Model file for the job. Use its own axes, mm. Face numbers are marked on the shaded views. A direction names the side the tool comes from. Coordinates: 2 decimals unless noted, no trailing zeros. Write each loop counter-clockwise with the first axis right and the second up, starting at its lowest first coordinate (ties: lowest second). Pieces come first, ordered by that corner, then holes. Notation, with made-up numbers: M 44,89.5 L 62,89.5 A23 cw 62,121.5 Z; hole C -18.5,9 d11. An arc over 180 degrees is marked long. Put each result on its own line as item: value. Start each with the question number.
Q1. Drop flat-ended pins along their axis: pin 1 (1.5 mm diameter, centred on y = 2, z = 4.5, fed in from +X); pin 2 (1.5 mm diameter, centred on y = -1, z = 6, fed in from -X); pin 3 (4 mm diameter, centred on x = 7.5, z = 5, fed in from +Y). Give the stop position or say it passes through.
Q2. Drill centre lines: line 1 along Y through (x, z) = (0, 3.75); line 2 along Y through (x, z) = (8.5, 6); line 3 along X through (y, z) = (0.75, 5). Where is each one in solid material? Low to high.
Q3. Cut at A-A (y = 0). Write the cut outline in (x, z), then the cut area to 3 significant figures.
Q4. Cut at D-D (y = 2.5). Write the cut outline in (x, z).
Q5. Cut at C-C (x = -0.75). Write the cut outline in (y, z).
Q6. Which spindle directions (+Z, -Z, +X, -X, +Y, -Y) get a long thin tool onto all of the face, cutting with end or side? Do the marked faces 1, 2 and 3. Say none if no direction does.
Q7. Cut at B-B (z = 6.25). Write the cut outline in (x, y).
```python
from build123d import *

# Parameters (mm, degrees)
CROQUIS1_R              = 4
CROQUIS1_R_2            = 2
SALIENTE_EXTRUIR1_DEPTH = 8
CROQUIS3_R              = 1.25
CORTAR_EXTRUIR1_DEPTH   = 21.5


with BuildPart() as part:
    # Croquis1 → Saliente-Extruir1 (new body)
    # profile 1 of 4: a face of its own
    with BuildSketch(Plane.XY):
        Circle(CROQUIS1_R)
        Circle(CROQUIS1_R_2, mode=Mode.SUBTRACT)
    # profile 2 of 4: a face of its own
    with BuildSketch(Plane.XY):
        with BuildLine():
            Line((8.464101615, 2), (3.464101615, 2))
            ThreePointArc((3.464101615, 2), (3.863703305, 1.03527618), (4, 0))
            ThreePointArc((4, 0), (3.863703305, -1.03527618), (3.464101615, -2))
            Line((3.464101615, -2), (8.464101615, -2))
            Line((8.464101615, -2), (8.464101615, 2))
        make_face()
    # profile 3 of 4: a face of its own
    with BuildSketch(Plane.XY):
        with BuildLine():
            Line((13.464101615, 2), (8.464101615, 2))
            Line((8.464101615, 2), (8.464101615, -2))
            Line((8.464101615, -2), (13.464101615, -2))
            ThreePointArc((13.464101615, -2), (12.92820323, 0), (13.464101615, 2))
        make_face()
    # profile 4 of 4: a face of its own
    with BuildSketch(Plane.XY):
        with Locations((16.92820323, 0)):
            Circle(CROQUIS1_R)
        with Locations((16.92820323, 0)):
            Circle(CROQUIS1_R_2, mode=Mode.SUBTRACT)
    extrude(amount=SALIENTE_EXTRUIR1_DEPTH)

    # Croquis3 → Cortar-Extruir1 (cut)
    with BuildSketch(Plane(origin=(0, 0, 0), x_dir=(-1, 0, 0), z_dir=(0, 0, -1))):
        with Locations((-8.464101615, 0)):
            Circle(CROQUIS3_R)
    extrude(amount=-CORTAR_EXTRUIR1_DEPTH, mode=Mode.SUBTRACT)


solid = part.part
```
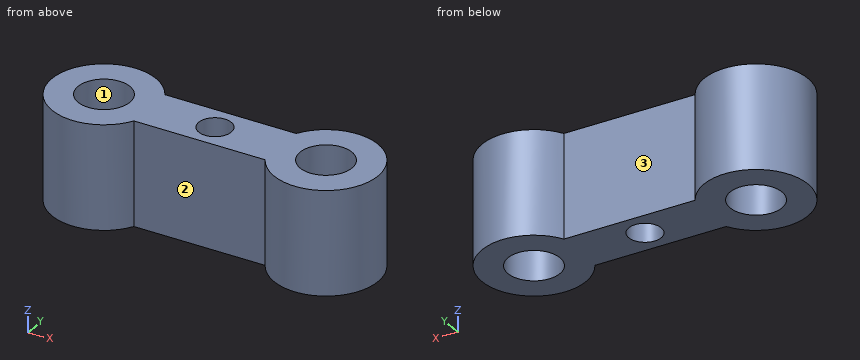
Computed values:
1. pin 1: x = 20.73
1. pin 2: x = -3.99
1. pin 3: y = 2
2. line 1: -4 to -2, 2 to 4
2. line 2: -2 to -1.25, 1.25 to 2
2. line 3: -3.93 to -1.85, 1.85 to 7.46, 9.46 to 15.07, 18.78 to 20.86
3. outline: M -4,0 L -2,0 L -2,8 L -4,8 Z; M 2,0 L 7.21,0 L 7.21,8 L 2,8 Z; M 9.71,0 L 14.93,0 L 14.93,8 L 9.71,8 Z; M 18.93,0 L 20.93,0 L 20.93,8 L 18.93,8 Z
3. area: 115 mm2
4. outline: M -3.12,0 L 3.12,0 L 3.12,8 L -3.12,8 Z; M 13.81,0 L 20.05,0 L 20.05,8 L 13.81,8 Z
5. outline: M -3.93,0 L -1.85,0 L -1.85,8 L -3.93,8 Z; M 1.85,0 L 3.93,0 L 3.93,8 L 1.85,8 Z
6. face 1: +Z, -Z
6. face 2: +Z, -Z, -Y
6. face 3: +Z, -Z, +Y
7. outline: M 3.46,-2 L 13.46,-2 A4 ccw long 13.46,2 L 3.46,2 A4 ccw long Z; hole C 0,0 d4; hole C 8.46,0 d2.5; hole C 16.93,0 d4
